```python
from build123d import *

# Parameters (mm, degrees)
F0_W     = 20
F0_H     = 32
F0_R     = 3.75
F1_DEPTH = 2
F2_DEPTH = 10
F3_DEPTH = 4


with BuildPart() as f1:
    # F0 (on Top) → F1 (new body)
    with BuildSketch(Plane.XY):
        Polygon((4, 18), (-4, 18), (-12, 18), (-12, 2), (-12, -2), (-12, -18), (-4, -18), (4, -18), (12, -18), (12, -2), (12, 2), (12, 18), align=None)
        Rectangle(F0_W, F0_H, mode=Mode.SUBTRACT)
        Rectangle(F0_W, F0_H)
        with BuildLine():
            Line((32.8394541729, -25), (12, -2))
            Line((12, -2), (12, -18))
            Line((12, -18), (4, -18))
            Line((4, -18), (26, -34.1306779105))
            ThreePointArc((26, -34.1306779105), (25.397931288, -26.552760007), (32.8394541729, -25))
        make_face()
        with BuildLine():
            Line((-12, -18), (-12, -2))
            Line((-12, -2), (-32.8394541729, -25))
            ThreePointArc((-32.8394541729, -25), (-27.1072816845, -25.0306257188), (-24.25, -30))
            ThreePointArc((-24.25, -30), (-24.7055453539, -32.2430448056), (-26, -34.1306779105))
            Line((-26, -34.1306779105), (-4, -18))
            Line((-4, -18), (-12, -18))
        make_face()
        with BuildLine():
            Line((26, 34.1306779105), (4, 18))
            Line((4, 18), (12, 18))
            Line((12, 18), (12, 2))
            Line((12, 2), (32.8394541729, 25))
            ThreePointArc((32.8394541729, 25), (25.397931288, 26.552760007), (26, 34.1306779105))
        make_face()
        with BuildLine():
            ThreePointArc((-26, 34.1306779105), (-24.7055453539, 32.2430448056), (-24.25, 30))
            ThreePointArc((-24.25, 30), (-27.1072816845, 25.0306257188), (-32.8394541729, 25))
            Line((-32.8394541729, 25), (-12, 2))
            Line((-12, 2), (-12, 18))
            Line((-12, 18), (-4, 18))
            Line((-4, 18), (-26, 34.1306779105))
        make_face()
        with BuildLine():
            ThreePointArc((35.75, -30), (34.9693742812, -27.1072816845), (32.8394541729, -25))
            ThreePointArc((32.8394541729, -25), (25.397931288, -26.552760007), (26, -34.1306779105))
            ThreePointArc((26, -34.1306779105), (32.2430448056, -35.2944546461), (35.75, -30))
        make_face()
        with Locations((30, -30)):
            Circle(F0_R, mode=Mode.SUBTRACT)
        with BuildLine():
            ThreePointArc((35.75, 30), (32.2430448056, 35.2944546461), (26, 34.1306779105))
            ThreePointArc((26, 34.1306779105), (25.397931288, 26.552760007), (32.8394541729, 25))
            ThreePointArc((32.8394541729, 25), (34.9693742812, 27.1072816845), (35.75, 30))
        make_face()
        with Locations((30, 30)):
            Circle(F0_R, mode=Mode.SUBTRACT)
        with BuildLine():
            ThreePointArc((-32.8394541729, 25), (-27.1072816845, 25.0306257188), (-24.25, 30))
            ThreePointArc((-24.25, 30), (-24.7055453539, 32.2430448056), (-26, 34.1306779105))
            ThreePointArc((-26, 34.1306779105), (-34.602068712, 33.447239993), (-32.8394541729, 25))
        make_face()
        with Locations((-30, 30)):
            Circle(F0_R, mode=Mode.SUBTRACT)
        with BuildLine():
            ThreePointArc((-24.25, -30), (-27.1072816845, -25.0306257188), (-32.8394541729, -25))
            ThreePointArc((-32.8394541729, -25), (-34.602068712, -33.447239993), (-26, -34.1306779105))
            ThreePointArc((-26, -34.1306779105), (-24.7055453539, -32.2430448056), (-24.25, -30))
        make_face()
        with Locations((-30, -30)):
            Circle(F0_R, mode=Mode.SUBTRACT)
    extrude(amount=F1_DEPTH)

    # F0 (on Top) → F2 (join)
    with BuildSketch(Plane.XY):
        with BuildLine():
            ThreePointArc((-32.8394541729, 25), (-27.1072816845, 25.0306257188), (-24.25, 30))
            ThreePointArc((-24.25, 30), (-24.7055453539, 32.2430448056), (-26, 34.1306779105))
            ThreePointArc((-26, 34.1306779105), (-34.602068712, 33.447239993), (-32.8394541729, 25))
        make_face()
        with Locations((-30, 30)):
            Circle(F0_R, mode=Mode.SUBTRACT)
        with BuildLine():
            ThreePointArc((35.75, -30), (34.9693742812, -27.1072816845), (32.8394541729, -25))
            ThreePointArc((32.8394541729, -25), (25.397931288, -26.552760007), (26, -34.1306779105))
            ThreePointArc((26, -34.1306779105), (32.2430448056, -35.2944546461), (35.75, -30))
        make_face()
        with Locations((30, -30)):
            Circle(F0_R, mode=Mode.SUBTRACT)
        with BuildLine():
            ThreePointArc((-24.25, -30), (-27.1072816845, -25.0306257188), (-32.8394541729, -25))
            ThreePointArc((-32.8394541729, -25), (-34.602068712, -33.447239993), (-26, -34.1306779105))
            ThreePointArc((-26, -34.1306779105), (-24.7055453539, -32.2430448056), (-24.25, -30))
        make_face()
        with Locations((-30, -30)):
            Circle(F0_R, mode=Mode.SUBTRACT)
        with BuildLine():
            ThreePointArc((35.75, 30), (32.2430448056, 35.2944546461), (26, 34.1306779105))
            ThreePointArc((26, 34.1306779105), (25.397931288, 26.552760007), (32.8394541729, 25))
            ThreePointArc((32.8394541729, 25), (34.9693742812, 27.1072816845), (35.75, 30))
        make_face()
        with Locations((30, 30)):
            Circle(F0_R, mode=Mode.SUBTRACT)
    extrude(amount=F2_DEPTH)

    # F0 (on Top) → F3 (join)
    with BuildSketch(Plane.XY):
        Polygon((4, 18), (-4, 18), (-12, 18), (-12, 2), (-12, -2), (-12, -18), (-4, -18), (4, -18), (12, -18), (12, -2), (12, 2), (12, 18), align=None)
        Rectangle(F0_W, F0_H, mode=Mode.SUBTRACT)
    extrude(amount=F3_DEPTH)


solid = f1.part
```
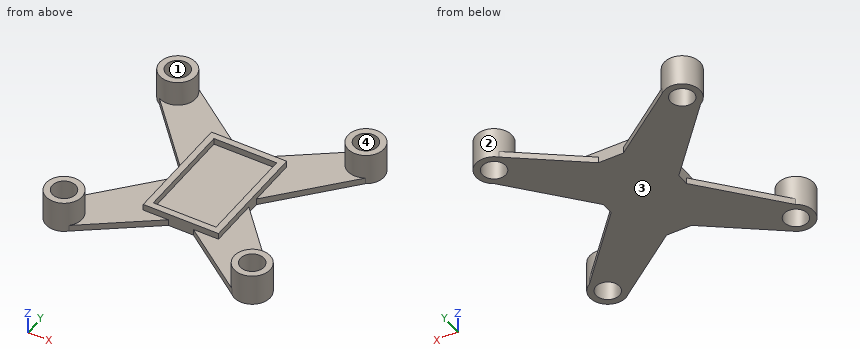
Geometry: final body of the model. Coordinates: model frame, mm. Face numbers are marked on the shaded views. A direction names the side the tool comes from. Round coordinates to 2 decimals unless told otherwise and drop trailing zeros. Write each loop counter-clockwise with the first axis right and the second up, starting at its lowest first coordinate (ties: lowest second). Pieces come first, ordered by that corner, then holes. Notation, with made-up numbers: M 43,-39.75 L 102,-39.75 A21 ccw 102,-14.75 Z; hole C -8,34.25 d1. An arc over 180 degrees is marked long. Answer in a Markdown table with one row per item. Add a question column.
(1) Cut plane A-A, the plane z = 8.75. Return the cut outline in (x, y), then the cut area to 3 significant figures.
(2) Contact query for flat-ended pins moving along their axis: pin 1 (4.5 mm diameter, centred on y = -1.5, z = 2.5, fed in from +X); pin 2 (8.5 mm diameter, centred on x = 13, y = -17, fed in from +Z); pin 3 (4 mm diameter, centred on x = 0, y = -13, fed in from +Z); pin 4 (8 mm diameter, centred on x = -21, y = 8.5, fed in from -Z). Output: stop coordinate, or through.
(3) Ray query, L1, parallel to Y at x = 30, z = 3; L2, parallel to X at y = 29, z = 5.25; L3, parallel to X at y = 6.5, z = 2.5. Return the intervals inside material, ascending.
(4) Cut plane C-C, the plane y = 30. Return the cut outline in (x, z), then the cut area to 3 significant figures.
(5) Cut plane D-D, the plane y = -21. Return the cut outline in (x, z), then the cut area to 3 significant figures.
(6) Cut plane B-B, the plane z = 3. Give the number of separate pieces and of enclosed holes in the cut face, then the cut area to 3 significant figures.
(7) Reachability of the marked faces 1 and 2 from +Z, -Z, +X, -X, +Y, -Y: full face, straight path, thin tool, end or side. Return the list, or none.
(8) Draft query along X for the marked faces 3 and 4. Return one class per face: pulls with the +X half, pulls with the -X half, needs draft (parallel to the pull), parting line crosses it, or undercut.
Established:
| question | item | result |
|---|---|---|
| 1 | outline | C -30,-30 d11.5; C -30,30 d11.5; C 30,-30 d11.5; C 30,30 d11.5; hole C -30,-30 d7.5; hole C -30,30 d7.5; hole C 30,-30 d7.5; hole C 30,30 d7.5 |
| 1 | area | 239 mm² |
| 2 | pin 1 | x = 13.53 |
| 2 | pin 2 | z = 4 |
| 2 | pin 3 | z = 2 |
| 2 | pin 4 | z = 0 |
| 3 | L1 | -35.75 to -33.75, -26.25 to -24.25, 24.25 to 26.25, 33.75 to 35.75 |
| 3 | L2 | -35.66 to -33.61, -26.39 to -24.34, 24.34 to 26.39, 33.61 to 35.66 |
| 3 | L3 | -12 to -10, 10 to 12 |
| 4 | outline | M -35.75,0 L -33.75,0 L -33.75,10 L -35.75,10 Z; M -26.25,0 L -20.37,0 L -20.37,2 L -24.25,2 L -24.25,10 L -26.25,10 Z; M 20.37,0 L 26.25,0 L 26.25,10 L 24.25,10 L 24.25,2 L 20.37,2 Z; M 33.75,0 L 35.75,0 L 35.75,10 L 33.75,10 Z |
| 4 | area | 95.5 mm² |
| 5 | outline | M -29.22,0 L -8.09,0 L -8.09,2 L -29.22,2 Z; M 8.09,0 L 29.22,0 L 29.22,2 L 8.09,2 Z |
| 5 | area | 84.5 mm² |
| 6 | separate pieces | 5 |
| 6 | enclosed holes | 5 |
| 6 | area | 463 mm² |
| 7 | face 1 | +Z, -Z |
| 7 | face 2 | +Z |
| 8 | face 3 | needs draft |
| 8 | face 4 | undercut |
